Verification items for the finished model (mm, model axes). Face numbers are marked on the shaded views. A direction names the side the tool comes from. Give positions to 0.01 mm unless a question says otherwise; leave off trailing zeros. Loops run counter-clockwise (first coordinate to the right, second up) from the corner with the lowest first, then second, coordinate; pieces in that order, holes last. Notation, with made-up numbers: M -27,21 L -15,21 A27 ccw -15,46 Z; hole C 86,39.25 d2. An arc over 180 degrees is marked long. Put each result on its own line as item: value. Start each with the question number.
from build123d import *

# Parameters (mm, degrees)
F1_DEPTH = 86
F2_W     = 160
F2_H     = 99
F3_DEPTH = 25
F4_R     = 15
F5_DEPTH = 25
F7_DEPTH = 2
F9_DEPTH = 2


with BuildPart() as f1:
    # F0 (on Right) → F1 (new body, symmetric)
    with BuildSketch(Plane.YZ):
        Polygon((63.122124, 2.497642), (17.160184, 48.459583), (-60.975116, -29.675717), (-60.975116, -99.675717), (63.122124, -99.675717), align=None)
        Polygon((61.122124, -97.675716), (-58.975115, -97.675716), (-58.975115, -30.504144), (17.160184, 45.631155), (61.122124, 1.669215), align=None, mode=Mode.SUBTRACT)
    extrude(amount=F1_DEPTH, both=True)

    # F2 (on face) → F3 (cut)
    with BuildSketch(Plane(origin=(0, -15.6497, 15.6497), x_dir=(1, 0, 0), z_dir=(0, -0.707107, 0.707107))):
        with Locations((0, -8.849818)):
            Rectangle(F2_W, F2_H)
    extrude(amount=-F3_DEPTH, mode=Mode.SUBTRACT)

    # F4 (on face) → F5 (cut)
    with BuildSketch(Plane(origin=(0, 63.122124, 0), x_dir=(-1, 0, 0), z_dir=(0, 1, 0))):
        with Locations((0, -64.675717)):
            Circle(F4_R)
    extrude(amount=-F5_DEPTH, mode=Mode.SUBTRACT)

    # F6 (on face) → F7 (join)
    with BuildSketch(Plane.YZ.offset(86)):
        Polygon((63.122124, 2.497642), (17.160184, 48.459583), (-60.975116, -29.675717), (-60.975116, -99.675717), (63.122124, -99.675717), align=None)
    extrude(amount=-F7_DEPTH)

    # F8 (on face) → F9 (join)
    with BuildSketch(Plane(origin=(-86, 0, 0), x_dir=(0, -1, 0), z_dir=(-1, 0, 0))):
        Polygon((-17.160184, 48.459583), (-63.122124, 2.497642), (-63.122124, -99.675717), (60.975116, -99.675717), (60.975116, -29.675717), align=None)
    extrude(amount=-F9_DEPTH)


solid = f1.part
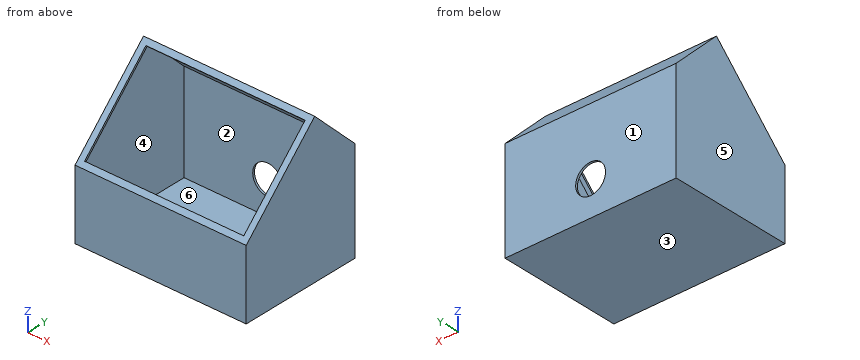
Q1. Scan lines: L1, parallel to X at y = 56, z = -81; L2, parallel to Y at x = 70.5, z = -48; L3, parallel to Z at x = -39, y = -18. Record each from-to range of solid material in increasing order.
Q2. Set-up check for the marked faces 1 and 2: record each of +Z, -Z, +X, -X, +Y, -Y from which the full face is reachable in a straight line by a thin tool's end or side.
Q3. Release check for a two-part mould opening along Z. For the marked faces 3, 4, 5 and 6 record: pulls with the +Z half, pulls with the -Z half, needs draft (parallel to the pull), parting line crosses it, or undercut.
Q4. Cross-section at D-D, the plane x = 27.5. Record the boundary of the cut face in (y, z).
Q5. Cross-section at A-A, the plane z = -90. Record the boundary of the cut face in (x, y).
Q6. Cross-section at B-B, the plane x = 0. Record the boundary of the cut face in (y, z).
Q7. Cross-section at C-C, the plane y = 48. Record the boundary of the cut face in (x, z), then the cut area to 3 significant figures.
Q8. Go/stop test with flat-tipped pins: pin 1 (5 mm diameter, centred on x = 45, z = 28, fed in from -Y); pin 2 (2 mm diameter, centred on x = -11.5, z = 28, fed in from -Y); pin 3 (6 mm diameter, centred on x = -40.5, y = -29, fed in from +Z). Record where each tip stops, or that it passes through.
Ans:
1. L1: x = -86 to -84, 84 to 86
1. L2: y = -60.98 to -58.98, 61.12 to 63.12
1. L3: z = -99.68 to -97.68
2. face 1: +Z, -Z, +X, -X, +Y
2. face 2: none
3. face 3: pulls with the -Z half
3. face 4: undercut
3. face 5: needs draft
3. face 6: undercut
4. outline: M -60.98,-99.68 L 63.12,-99.68 L 63.12,2.5 L 17.16,48.46 L 13.09,44.39 L 14.51,42.98 L 17.16,45.63 L 61.12,1.67 L 61.12,-97.68 L -58.98,-97.68 L -58.98,-30.5 L -55.5,-27.02 L -56.91,-25.61 L -60.98,-29.68 Z
5. outline: M -86,-60.98 L 86,-60.98 L 86,63.12 L -86,63.12 Z; hole M -84,-58.98 L 84,-58.98 L 84,61.12 L -84,61.12 Z
6. outline: M -60.98,-99.68 L 63.12,-99.68 L 63.12,-79.68 L 61.12,-79.68 L 61.12,-97.68 L -58.98,-97.68 L -58.98,-30.5 L -55.5,-27.02 L -56.91,-25.61 L -60.98,-29.68 Z; M 13.09,44.39 L 14.51,42.98 L 17.16,45.63 L 61.12,1.67 L 61.12,-49.68 L 63.12,-49.68 L 63.12,2.5 L 17.16,48.46 Z
7. outline: M -86,-99.68 L 86,-99.68 L 86,17.62 L -86,17.62 Z; hole M -84,-97.68 L 84,-97.68 L 84,14.79 L -84,14.79 Z
7. area: 1,280 mm^2
8. pin 1: stops at y = 32.29
8. pin 2: stops at y = 33.79
8. pin 3: stops at z = -97.68
